Part model, mm, in its own coordinate system. Face numbers are marked on the shaded views. A direction names the side the tool comes from. Give positions to 0.01 mm unless a question says otherwise; leave off trailing zeros. Write each loop counter-clockwise with the first axis right and the second up, starting at its lowest first coordinate (ties: lowest second). Pieces come first, ordered by that corner, then holes.
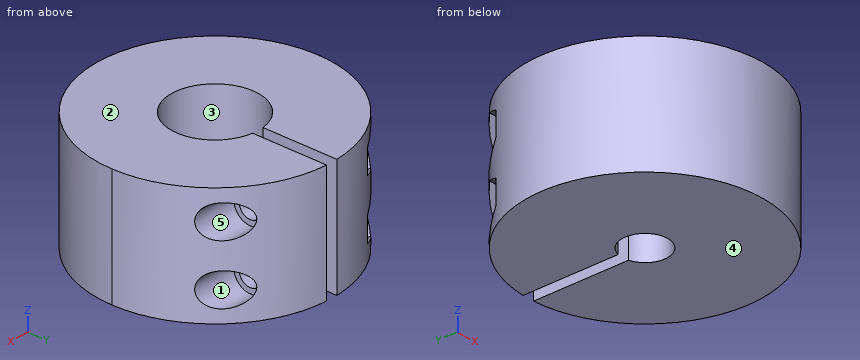
```python
from build123d import *

# Parameters (mm, degrees)
SKETCH1_R                       = 25.4
BOSS_EXTRUDE1_DEPTH             = 25.4
SKETCH2_R                       = 4.8895
CUT_EXTRUDE1_DEPTH              = 11.43
SKETCH3_R                       = 9.398
CUT_EXTRUDE2_DEPTH              = 13.97
DIVIDE_REACH                    = 45.994
SKETCH7_W                       = 2.54
SKETCH7_H                       = 25.4
SKETCH8_R                       = 2.413
F_4_40_THROUGH_HOLE_DEPTH       = 45.739343983
SKETCH9_R                       = 3.556
F_4_40_HEAD_CLEARANCE_DEPTH     = 52.446758086
F_4_40_HEX_NUT_DEPRESSION_DEPTH = 52.446758086
LPATTERN1_COUNT                 = 2
LPATTERN1_PITCH                 = 12.7


with BuildPart() as part:
    # Sketch1 → Boss-Extrude1 (new body)
    with BuildSketch(Plane.XY):
        Circle(SKETCH1_R)
    extrude(amount=BOSS_EXTRUDE1_DEPTH)

    # Sketch2 → Cut-Extrude1 (cut)
    with BuildSketch(Plane(origin=(0, 0, 0), x_dir=(-1, 0, 0), z_dir=(0, 0, -1))):
        Circle(SKETCH2_R)
    extrude(amount=-CUT_EXTRUDE1_DEPTH, mode=Mode.SUBTRACT)

    # Sketch3 → Cut-Extrude2 (cut)
    with BuildSketch(Plane.XY.offset(25.4)):
        Circle(SKETCH3_R)
    extrude(amount=-CUT_EXTRUDE2_DEPTH, mode=Mode.SUBTRACT)

    # Sketch7 → Divide (cut, up to next)
    with BuildSketch(Plane(origin=(0, 0, 0), x_dir=(-1, 0, 0), z_dir=(0, 0, -1)), mode=Mode.PRIVATE) as divide_sk1:
        with Locations((0, 12.7)):
            Rectangle(SKETCH7_W, SKETCH7_H)
    divide_tool1 = extrude(divide_sk1.sketch, amount=-DIVIDE_REACH, mode=Mode.PRIVATE) & part.part
    add(divide_tool1.solids().sort_by_distance((0, 12.7, 0))[0], mode=Mode.SUBTRACT)

    # Sketch8 → 4-40 through hole (cut, symmetric)
    with BuildSketch(Plane.ZY.offset(-1.27)):
        with Locations((19.05, 17.748230131)):
            Circle(SKETCH8_R)
    f_4_40_through_hole = extrude(amount=F_4_40_THROUGH_HOLE_DEPTH, both=True, mode=Mode.SUBTRACT)

    # Sketch9 → 4-40 head clearance (cut, through all)
    with BuildSketch(Plane.ZY.offset(-11.43)):
        with Locations((19.05, 17.748230131)):
            Circle(SKETCH9_R)
    f_4_40_head_clearance = extrude(amount=-F_4_40_HEAD_CLEARANCE_DEPTH, mode=Mode.SUBTRACT)

    # Sketch10 → 4-40 hex nut depression (cut, through all)
    with BuildSketch(Plane(origin=(-11.43, 0, 0), x_dir=(0, 0, -1), z_dir=(1, 0, 0))):
        Polygon((-21.616321947, 13.303230131), (-16.483678053, 13.303230131), (-13.917356107, 17.748230131), (-16.483678053, 22.193230131), (-21.616321947, 22.193230131), (-24.182643893, 17.748230131), align=None)
    f_4_40_hex_nut_depression = extrude(amount=-F_4_40_HEX_NUT_DEPRESSION_DEPTH, mode=Mode.SUBTRACT)

    # LPattern1: 4-40 through hole, 4-40 head clearance, 4-40 hex nut depression ×2
    with Locations(*[(0, 0, -i * LPATTERN1_PITCH) for i in range(1, LPATTERN1_COUNT)]):
        add(f_4_40_through_hole, mode=Mode.SUBTRACT)
        add(f_4_40_head_clearance, mode=Mode.SUBTRACT)
        add(f_4_40_hex_nut_depression, mode=Mode.SUBTRACT)


solid = part.part
```
1) Saw through at D-D, the plane z = 6.35. Write the cut outline in (x, y), then the cut area to 3 significant figures.
Answers follow:
outline: (-21.64, 13.3) arc R25.4 ccw (long way) to (21.07, 14.19) - (11.43, 14.19) - (11.43, 15.34) - (1.27, 15.34) - (1.27, 4.72) arc R4.89 cw (long way) to (-1.27, 4.72) - (-1.27, 15.34) - (-11.43, 15.34) - (-11.43, 13.3) - close; (-12.35, 22.19) - (-11.43, 22.19) - (-11.43, 20.16) - (-1.27, 20.16) - (-1.27, 25.37) arc R25.4 ccw to start; (1.27, 20.16) - (11.43, 20.16) - (11.43, 21.3) - (13.83, 21.3) arc R25.4 ccw to (1.27, 25.37) - close
area: 1,700 mm2
2) Saw through at B-B, the plane x = -3. Write the cut outline in (y, z), then the cut area to 3 significant figures.
Answers follow:
outline: (-25.22, 0) - (-3.86, 0) - (-3.86, 11.43) - (-8.91, 11.43) - (-8.91, 25.4) - (-25.22, 25.4) - close; (3.86, 0) - (25.22, 0) - (25.22, 25.4) - (8.91, 25.4) - (8.91, 11.43) - (3.86, 11.43) - close; hole circle Ø4.83 at (17.75, 6.35); hole circle Ø4.83 at (17.75, 19.05)
area: 908 mm2
3) Wall check: L1, parallel to X at y = 0, z = 3; L2, parallel to Y at x = 6, z = 19.05; L3, parallel to X at y = 20.5, z = 5.5. Give the ranges that are in metal, low to high.
Answers follow:
L1: x = -25.4 to -4.89, 4.89 to 25.4
L2: y = -24.68 to -7.23, 7.23 to 15.34, 20.16 to 24.68
L3: x = -11.43 to -1.27, 1.27 to 11.43
4) Two-plate mould, pull along Y, no slides. Class the marked faces 1 and 2: +Y half, -Y half, draft (parallel to the pull), parting line (faces both ways), or undercut.
Answers follow:
face 1: undercut
face 2: draft
5) Saw through at A-A, the plane z = 20.5. Write the cut outline in (x, y), then the cut area to 3 significant figures.
Answers follow:
outline: (-21.64, 13.3) arc R25.4 ccw (long way) to (20.85, 14.5) - (11.43, 14.5) - (11.43, 15.82) - (1.27, 15.82) - (1.27, 9.31) arc R9.4 cw (long way) to (-1.27, 9.31) - (-1.27, 15.82) - (-11.43, 15.82) - (-11.43, 13.3) - close; (-12.35, 22.19) - (-11.43, 22.19) - (-11.43, 19.68) - (-1.27, 19.68) - (-1.27, 25.37) arc R25.4 ccw to start; (1.27, 19.68) - (11.43, 19.68) - (11.43, 21) - (14.3, 21) arc R25.4 ccw to (1.27, 25.37) - close
area: 1,530 mm2
6) 3-axis set-ups, long thin cutter, end or side, ignore diameter. For the marked faces 3, 4 and 5: which of +Z, -Z, +X, -X, +Y, -Y reach the whole face in a straight line?
Answers follow:
face 3: +Z
face 4: -Z, +X, -X, +Y, -Y
face 5: +X
7) Saw through at C-C, the plane y = -19.5. Write the cut outline in (x, z), then the cut area to 3 significant figures.
Answers follow:
outline: (-16.28, 0) - (16.28, 0) - (16.28, 25.4) - (-16.28, 25.4) - close
area: 827 mm2
8) Pin check, flat tips, straight feed: pin 1 Ø8 at (y, z) = (-5, 19.5) entering from -X; pin 2 Ø2.5 at (y, z) = (19.5, 5.5) entering from -X; pin 3 Ø10 at (y, z) = (16.5, 19.5) entering from -X. Stop position of each tip, or through.
Answers follow:
pin 1: stops at x = -25.38
pin 2: stops at x = -11.43
pin 3: stops at x = -22.65
